Build history of the part. All positions in model axes, mm. A direction names the side the tool comes from. Round coordinates to 2 decimals unless told otherwise and drop trailing zeros. Loops run counter-clockwise (first coordinate to the right, second up) from the corner with the lowest first, then second, coordinate; pieces in that order, holes last. Notation, with made-up numbers: (51, 17.5) -> (71, 17.5) arc R30 ccw to (71, 46.5) -> close; hole circle Ø5 at (15.25, 53). An arc over 180 degrees is marked (long way). Put each result on its own line as item: value. Start each with the question number.
Item 1: Cut at B-B, the plane y = -23.5. List the corners of the cut face in (x, z), plus the area to 3 significant figures.
Item 2: Cut at C-C, the plane z = -108.5. List the corners of the cut face in (x, y).
Item 3: Tool access for faces 4 (the flat face through (-69.85, -100, -67)), 5 (the flat face through (105, -127, -7.938)), 6 (the flat face through (-2, -253, -50.8)), 7 (the flat face through (-106, -127, -7.938)): list every direction of +Z, -Z, +X, -X, +Y, -Y with a clear straight run to the whole face (end or side of a thin tool).
Item 4: Cut at A-A, the plane x = -15. List the corners of the cut face in (y, z) (1 decimal).
Item 5: Flat gauge pins, fed straight in: pin 1 Ø6 at (x, z) = (-52.5, -89) entering from -Y; pin 2 Ø6 at (x, y) = (-89.5, -199.5) entering from -Z; pin 3 Ø6.5 at (x, y) = (-63.5, -251.5) entering from -Z. Where does each tip first touch, or does it go through?
Item 6: Pull direction Y, two halves, no side cores. Call faces 1 (the flat face through (-2, -257.175, -25)), 2 (the flat face through (69.85, -100, -65)), 3 (the flat face through (-133.35, -90, -3)): +Y half, -Y half, draft (parallel to the pull), parting line (faces both ways), or undercut.
Item 7: Drill centre lines: probe 1 along Y at (x, z) = (15.5, -49.5) (1 decimal); probe 2 along X at (y, z) = (-161.5, -10); probe 3 along Z at (x, y) = (-91.5, -49.5). Where is each one in solid material? Low to high. Write a range as [from, to].
```python
from build123d import *

# Parameters (mm, degrees)
F0_W     = 266.7
F0_H     = 158.12516
F1_DEPTH = 7.9375
F4_DEPTH = 241.3
F6_DEPTH = 211.1385
F8_W     = 266.7
F8_H     = 50.8
F9_DEPTH = 7.9375


with BuildPart() as f1:
    # F0 (on Front) → F1 (new body)
    with BuildSketch(Plane.XZ):
        with Locations((0, -79.06258)):
            Rectangle(F0_W, F0_H)
    extrude(amount=F1_DEPTH)

    # F3 (on face) → F4 (join)
    with BuildSketch(Plane.XZ.offset(7.9375)):
        Polygon((133.35, 0), (-133.35, 0), (-133.35, -7.9375), (-77.7875, -7.9375), (-77.7875, -158.12516), (-69.85, -158.12516), (-69.85, -7.9375), (69.85, -7.9375), (69.85, -158.12516), (77.7875, -158.12516), (77.7875, -7.9375), (133.35, -7.9375), align=None)
    extrude(amount=F4_DEPTH)

    # F5 (on face) → F6 (cut, through all)
    with BuildSketch(Plane(origin=(-77.7875, 0, 0), x_dir=(0, -1, 0), z_dir=(-1, 0, 0))):
        Polygon((249.2375, -50.8), (46.0375, -158.12516), (249.2375, -158.12516), align=None)
    extrude(amount=-F6_DEPTH, mode=Mode.SUBTRACT)

    # F8 (on face) → F9 (join)
    with BuildSketch(Plane.XZ.offset(249.2375)):
        with Locations((0, -25.4)):
            Rectangle(F8_W, F8_H)
    extrude(amount=F9_DEPTH)


solid = f1.part
```
Reply:
1. outline: (-133.35, -7.94) -> (-77.79, -7.94) -> (-77.79, -158.13) -> (-69.85, -158.13) -> (-69.85, -7.94) -> (69.85, -7.94) -> (69.85, -158.13) -> (77.79, -158.13) -> (77.79, -7.94) -> (133.35, -7.94) -> (133.35, 0) -> (-133.35, 0) -> close
1. area: 4,500 mm^2
2. outline: (-133.35, -7.94) -> (-77.79, -7.94) -> (-77.79, -139.99) -> (-69.85, -139.99) -> (-69.85, -7.94) -> (69.85, -7.94) -> (69.85, -139.99) -> (77.79, -139.99) -> (77.79, -7.94) -> (133.35, -7.94) -> (133.35, 0) -> (-133.35, 0) -> close
3. face 4: -Z
3. face 5: -Z, +X
3. face 6: -Z, +X, -X, -Y
3. face 7: -Z, -X
4. outline: (-257.2, -50.8) -> (-249.2, -50.8) -> (-249.2, -7.9) -> (-7.9, -7.9) -> (-7.9, -158.1) -> (0, -158.1) -> (0, 0) -> (-257.2, 0) -> close
5. pin 1: stops at y = -7.94
5. pin 2: stops at z = -7.94
5. pin 3: stops at z = -50.8
6. face 1: -Y half
6. face 2: undercut
6. face 3: draft
7. probe 1: y = [-257.2, -249.2], [-7.9, 0]
7. probe 2: x = [-77.79, -69.85], [69.85, 77.79]
7. probe 3: z = [-7.94, 0]
